Could you check a few things on this model? Use its own coordinates, in mm. A direction names the side the tool comes from. Give positions to 0.01 mm unless a question says otherwise; leave off trailing zeros. Loops run counter-clockwise (first coordinate to the right, second up) from the corner with the lowest first, then second, coordinate; pieces in that order, holes last. Notation, with made-up numbers: (77.25, 2.25) - (132.25, 2.25) arc R26 cw to (132.25, 25.25) - close; hole circle Ø8 at (-29, 79.25). An arc over 180 degrees is marked (long way). Write each question's results on one line, items separated by ' | '. Start each with the question number.
```python
from build123d import *

# Parameters (mm, degrees)
BOSS_EXTRUDE1_DEPTH = 1.6
BOSS_EXTRUDE2_DEPTH = 15.4
SKETCH3_R           = 1.7
CUT_EXTRUDE1_DEPTH  = 1.6


with BuildPart() as part:
    # Sketch1 → Boss-Extrude1 (new body)
    with BuildSketch(Plane(origin=(0, 0, 0), x_dir=(1, 0, 0), z_dir=(0, 1, 0))):
        with BuildLine():
            Line((-24, -16), (24, -16))
            ThreePointArc((24, -16), (25.414213562, -15.414213562), (26, -14))
            Line((26, -14), (26, 14))
            ThreePointArc((26, 14), (25.414213562, 15.414213562), (24, 16))
            Line((24, 16), (-24, 16))
            ThreePointArc((-24, 16), (-25.414213562, 15.414213562), (-26, 14))
            Line((-26, 14), (-26, -14))
            ThreePointArc((-26, -14), (-25.414213562, -15.414213562), (-24, -16))
        make_face()
    extrude(amount=BOSS_EXTRUDE1_DEPTH)

    # Sketch2 → Boss-Extrude2 (add)
    with BuildSketch(Plane(origin=(0, 1.6, 0), x_dir=(1, 0, 0), z_dir=(0, 1, 0))):
        with BuildLine():
            Line((-18, -12.5), (18, -12.5))
            ThreePointArc((18, -12.5), (19.414213562, -11.914213562), (20, -10.5))
            Line((20, -10.5), (20, 10.5))
            ThreePointArc((20, 10.5), (19.414213562, 11.914213562), (18, 12.5))
            Line((18, 12.5), (-18, 12.5))
            ThreePointArc((-18, 12.5), (-19.414213562, 11.914213562), (-20, 10.5))
            Line((-20, 10.5), (-20, -10.5))
            ThreePointArc((-20, -10.5), (-19.414213562, -11.914213562), (-18, -12.5))
        make_face()
    extrude(amount=BOSS_EXTRUDE2_DEPTH)

    # Sketch3 → Cut-Extrude1 (cut)
    with BuildSketch(Plane(origin=(0, 0, 0), x_dir=(1, 0, 0), z_dir=(0, 1, 0))):
        with Locations(Location((22.5, -12.5, 0), (0, 0, 270))):
            Circle(SKETCH3_R)
        with Locations(Location((22.5, 12.5, 0), (0, 0, 270))):
            Circle(SKETCH3_R)
        with Locations(Location((-22.5, -12.5, 0), (0, 0, 270))):
            Circle(SKETCH3_R)
        with Locations(Location((-22.5, 12.5, 0), (0, 0, 270))):
            Circle(SKETCH3_R)
    extrude(amount=CUT_EXTRUDE1_DEPTH, mode=Mode.SUBTRACT)


solid = part.part
```
Q1. Which directions (+Z, -Z, +X, -X, +Y, -Y) give clear straight access to the entire face, cutting with the end or side of a thin tool? Please do faces 1 (the face through (0, 9, -12.5)), 2 (the face through (-20, 9, 0)), 3 (the face through (0, 9, 12.5)), 4 (the face through (19.43, 9.19, -11.9)).
Q2. I want a section at D-D, the plane z = -5.5. List the corners of the cut face in (x, y) for me.
Q3. I'm going to push flat-ended pins straight in: pin 1 Ø4.5 at (x, y) = (-8, 6.5) entering from -Z; pin 2 Ø8 at (y, z) = (5, 10) entering from -X; pin 3 Ø1.5 at (y, z) = (9.5, -4) entering from -X; pin 4 Ø1 at (x, y) = (5.5, 6) entering from +Z. Where does each tip first touch, or does it pass through?
Q4. I need wall thicknesses on L1, parallel to X at y = 0.6, z = -12.5; L2, parallel to X at y = 13.5, z = 5; L3, parallel to Z at x = -13, y = 15.5. Which ranges of each line are inside material? Lowest first, please. Write a range as from..to.
Q5. I want a section at C-C, the plane y = 9. List the corners of the cut face in (x, z) for me.
Q6. If we mould it in two halves opening along Z, with no side actions, what happens to faces 5 (the face through (25.43, 0.79, -15.4)), 6 (the face through (19.4, 9.19, 11.93)), 7 (the face through (-21.99, 0.79, -10.88))? For each: +Z half, -Z half, draft (parallel to the pull), parting line (faces both ways), or undercut.
Q7. I want a section at B-B, the plane z = 11.5. List the corners of the cut face in (x, y) for me.
Q8. I want a section at A-A, the plane x = -22.5. List the corners of the cut face in (y, z) for me.
Conclusion:
1) face 1: -Z, +X, -X, +Y | face 2: +Z, -Z, -X, +Y | face 3: +Z, +X, -X, +Y | face 4: -Z, +X, +Y
2) outline: (-26, 0) - (26, 0) - (26, 1.6) - (20, 1.6) - (20, 17) - (-20, 17) - (-20, 1.6) - (-26, 1.6) - close
3) pin 1: z = -12.5 | pin 2: x = -26 | pin 3: x = -20 | pin 4: z = 12.5
4) L1: -26..-24.2, -20.8..20.8, 24.2..26 | L2: -20..20 | L3: -12.5..12.5
5) outline: (-20, -10.5) arc R2 ccw to (-18, -12.5) - (18, -12.5) arc R2 ccw to (20, -10.5) - (20, 10.5) arc R2 ccw to (18, 12.5) - (-18, 12.5) arc R2 ccw to (-20, 10.5) - close
6) face 5: -Z half | face 6: +Z half | face 7: undercut
7) outline: (-26, 0) - (-23.87, 0) - (-23.87, 1.6) - (-26, 1.6) - close; (-21.13, 0) - (21.13, 0) - (21.13, 1.6) - (19.73, 1.6) - (19.73, 17) - (-19.73, 17) - (-19.73, 1.6) - (-21.13, 1.6) - close; (23.87, 0) - (26, 0) - (26, 1.6) - (23.87, 1.6) - close
8) outline: (0, -16) - (1.6, -16) - (1.6, -14.2) - (0, -14.2) - close; (0, -10.8) - (1.6, -10.8) - (1.6, 10.8) - (0, 10.8) - close; (0, 14.2) - (1.6, 14.2) - (1.6, 16) - (0, 16) - close
